Geometry: final body of the model. Coordinates: model frame, mm. A direction names the side the tool comes from. Coordinates: 2 decimals unless noted, no trailing zeros. Order: outer loops, then holes, each group sorted by start corner. A loop starts at its lowest first (then second) coordinate and runs counter-clockwise, first axis right, second up. Notation, with made-up numbers: M 47,-33 L 66,-33 A27 ccw 66,-1 Z; hole C 46,-29 d11. An arc over 180 degrees is marked long. Write item = value, one per line.
from build123d import *

# Parameters (mm, degrees)
F1_DEPTH  = 52
F2_W      = 9
F2_H      = 9
F3_DEPTH  = 2
F5_W      = 9
F5_H      = 7
F6_DEPTH  = 2
F7_W      = 9
F7_H      = 7
F8_DEPTH  = 2
F4_W      = 5
F4_H      = 17.54
F9_DEPTH  = 7
F10_W     = 5
F10_H     = 6.5
F10_H_2   = 6.04
F11_DEPTH = 51.001


with BuildPart() as f1:
    # F0 (on Front) → F1 (new body)
    with BuildSketch(Plane.XZ):
        Polygon((31.5, 0), (0, 0), (0, 13.54), (29.5, 13.54), (29.5, 10.54), (31.5, 10.54), (31.5, 15.54), (-2, 15.54), (-2, -2), (31.5, -2), align=None)
    extrude(amount=F1_DEPTH)

    # F2 (on face) → F3 (cut, through all)
    with BuildSketch(Plane(origin=(-2, 0, 0), x_dir=(0, -1, 0), z_dir=(-1, 0, 0))):
        with Locations((25.7, 9.04)):
            Rectangle(F2_W, F2_H)
    extrude(amount=-F3_DEPTH, mode=Mode.SUBTRACT)

    # F5 (on face) → F6 (join)
    with BuildSketch(Plane(origin=(0, 0, 0), x_dir=(-1, 0, 0), z_dir=(0, 1, 0))):
        with Locations((-2.5, 12.04)):
            Rectangle(F5_W, F5_H)
    extrude(amount=F6_DEPTH)

    # F7 (on face) → F8 (join)
    with BuildSketch(Plane.XZ.offset(52)):
        with Locations((2.5, 12.04)):
            Rectangle(F7_W, F7_H)
    extrude(amount=F8_DEPTH)

    # F4 (on face) → F9 (join)
    with BuildSketch(Plane(origin=(-2, 0, 0), x_dir=(0, -1, 0), z_dir=(-1, 0, 0))):
        with Locations((15.5, 6.77)):
            Rectangle(F4_W, F4_H)
        with Locations((5.5, 6.77)):
            Rectangle(F4_W, F4_H)
        with Locations((36.5, 6.77)):
            Rectangle(F4_W, F4_H)
        with Locations((46.5, 6.77)):
            Rectangle(F4_W, F4_H)
    extrude(amount=F9_DEPTH)

    # F10 (on face) → F11 (cut, through all)
    with BuildSketch(Plane(origin=(0, -3, 0), x_dir=(-1, 0, 0), z_dir=(0, 1, 0))):
        with Locations((4.5, 10.79)):
            Rectangle(F10_W, F10_H)
        with Locations((4.5, 3.02)):
            Rectangle(F10_W, F10_H_2)
    extrude(amount=-F11_DEPTH, mode=Mode.SUBTRACT)


solid = f1.part
1) Section D-D, the plane z = 6.75. Return loops of the section in (x, y), and give its area (3 significant figures).
Numbers:
outline = M -9,-49 L -2,-49 L -2,-52 L 0,-52 L 0,-30.2 L -2,-30.2 L -2,-34 L -9,-34 L -9,-39 L -2,-39 L -2,-44 L -9,-44 Z; M -9,-18 L -2,-18 L -2,-21.2 L 0,-21.2 L 0,0 L -2,0 L -2,-3 L -9,-3 L -9,-8 L -2,-8 L -2,-13 L -9,-13 Z
area = 226 mm²
2) Section B-B, the plane y = -22. Return loops of the section in (x, z), and give its area (3 significant figures).
Numbers:
outline = M -2,-2 L 31.5,-2 L 31.5,0 L 0,0 L 0,4.54 L -2,4.54 Z; M -2,13.54 L 29.5,13.54 L 29.5,10.54 L 31.5,10.54 L 31.5,15.54 L -2,15.54 Z
area = 149 mm²
3) Mould query, pull axis Y, two halves, no side actions, for faces 4 (the face through (3, 2, 12)), 5 (the face through (7, -53, 12)), 6 (the face through (3, -52, 11)). Classes: pulls with the +Y half, pulls with the -Y half, needs draft (parallel to the pull), parting line crosses it, or undercut.
Numbers:
face_4 = pulls with the +Y half
face_5 = needs draft
face_6 = undercut
4) Set-up query: faces 1 (the face through (2, -53, 8.54)), 2 (the face through (-6, -13, 7)), 3 (the face through (-7, -15, 3)). Return all of +Z, -Z, +X, -X, +Y, -Y with unobstructed straight access to the full face (end or side cutting, diameter ignored); none if empty.
Numbers:
face_1 = -Z, +X, -X, -Y
face_2 = +Z, -Z, -X
face_3 = +Y, -Y
5) Pin query (flat end, axial travel): pin 1 (2 mm diameter, centred on x = -4.5, z = 7, fed in from +Y); pin 2 (2 mm diameter, centred on x = -1, z = 7, fed in from -Y); pin 3 (2.5 mm diameter, centred on y = -29.5, z = 11.5, fed in from -X). Return the tip coordinate at first contact, or that it passes through.
Numbers:
pin_1 = -3
pin_2 = -52
pin_3 = -2
6) Section A-A, the plane z = 2.5. Return loops of the section in (x, y).
Numbers:
outline = M -9,-49 L -7,-49 L -7,-44 L -9,-44 Z; M -9,-39 L -7,-39 L -7,-34 L -9,-34 Z; M -9,-18 L -7,-18 L -7,-13 L -9,-13 Z; M -9,-8 L -7,-8 L -7,-3 L -9,-3 Z; M -2,-52 L 0,-52 L 0,0 L -2,0 Z
7) Line query: L1, parallel to Y at x = -5, z = 6.5; L2, parallel to Z at x = 13, y = -11.5; L3, parallel to X at y = -18.5, z = 13. Output: solid intervals per line, ascending.
Numbers:
L1 = -49 to -44, -39 to -34, -18 to -13, -8 to -3
L2 = -2 to 0, 13.54 to 15.54
L3 = -2 to 0, 29.5 to 31.5
8) Section C-C, the plane x = 3. Return loops of the section in (y, z), and give its area (3 significant figures).
Numbers:
outline = M -54,8.54 L -52,8.54 L -52,13.54 L 0,13.54 L 0,8.54 L 2,8.54 L 2,15.54 L -54,15.54 Z; M -52,-2 L 0,-2 L 0,0 L -52,0 Z
area = 236 mm²
